CAD build for the part. Positions are in the model's coordinates, mm. Face numbers are marked on the shaded views. Round coordinates to 2 decimals unless told otherwise and drop trailing zeros. Write each loop counter-clockwise with the first axis right and the second up, starting at its lowest first coordinate (ties: lowest second). Pieces come first, ordered by that corner, then holes. Notation, with made-up numbers: (-30, 73) -> (25, 73) arc R28 ccw to (25, 100) -> close; hole circle Ø4 at (43, 33.5). An arc over 180 degrees is marked (long way). Put each result on its own line as item: value. Start each with the question number.
1. Saw through at D-D on x = 3.5. List the corners of the cut face in (y, z).
2. Drill centre lines: line 1 (Z direction, x = 5.9, y = 0); line 2 (Z direction, x = 3.75, y = -1.5); line 3 (X direction, y = -6, z = -15). Where is each one in solid material? Low to high. Write a range as from..to.
3. Pull direction Z, two halves, no side cores. Call the marked faces 1, 2 and 3: pulls with the +Z half, pulls with the -Z half, needs draft (parallel to the pull), parting line crosses it, or undercut.
4. Flat gauge pins, fed straight in: P1, Ø2, axis at x = 3, y = -5, coming from the -Z side; P2, Ø2, axis at x = 1, z = -3, coming from the +Y side. Where does each tip first touch, or does it go through?
5. Saw through at A-A on y = 0. List the corners of the cut face in (x, z).
6. Saw through at C-C on x = 1.5. List the corners of the cut face in (y, z).
from build123d import *


with BuildPart() as part:
    # 草图1 → 旋转1 (revolve)
    with BuildSketch(Plane.XY):
        with BuildLine():
            Line((5.6, 5.1), (5.6, 4))
            Line((5.6, 4), (6.5, 4))
            Line((6.5, 4), (6.5, 10))
            Line((6.5, 10), (6, 12))
            Line((6, 12), (6, 17))
            Line((6, 17), (5, 17))
            ThreePointArc((5, 17), (3, 14.990135067), (1, 17))
            Line((1, 17), (0, 17))
            Line((0, 17), (0, 5.1))
            Line((0, 5.1), (5.6, 5.1))
        make_face()
    revolve(axis=Axis((0, 0, 0), (1, 0, 0)))


solid = part.part
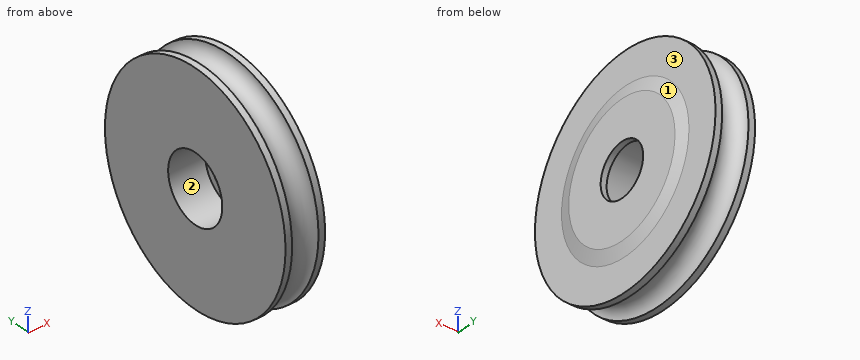
Return value:
1. outline: circle Ø30.11 at (0, 0); hole circle Ø10.2 at (0, 0)
2. line 1: z = -17..-4, 4..17
2. line 2: z = -15.06..-4.87, 4.87..15.06
2. line 3: x = 0..1.18, 4.82..6
3. face 1: parting line crosses it
3. face 2: undercut
3. face 3: needs draft
4. P1: stops at z = -14.51
4. P2: stops at y = 16.88
5. outline: (0, -17) -> (1, -17) arc R2 cw (long way) to (5, -17) -> (6, -17) -> (6, -12) -> (6.5, -10) -> (6.5, -4) -> (5.6, -4) -> (5.6, -5.1) -> (0, -5.1) -> close; (0, 5.1) -> (5.6, 5.1) -> (5.6, 4) -> (6.5, 4) -> (6.5, 10) -> (6, 12) -> (6, 17) -> (5, 17) arc R2 cw (long way) to (1, 17) -> (0, 17) -> close
6. outline: circle Ø31.33 at (0, 0); hole circle Ø10.2 at (0, 0)
